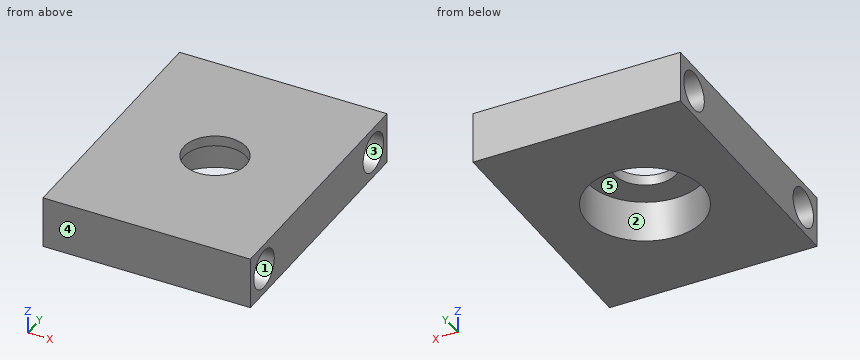
Autodesk Fusion 360 part; units mm, degrees
sketch "Top" plane through (0, 0, 0) normal (0, 0, 1) x (1, 0, 0)
  line L0 (0, 0) -> (40, 0)
  line L1 (40, 0) -> (40, 50)
  line L2 (40, 50) -> (0, 50)
  line L3 (0, 50) -> (0, 0)
  circle A0 centre (20, 25) radius 11.2
  circle A1 centre (20, 25) radius 6
  dimension "d6" = 40
  dimension "d7" = 50
  dimension "d11" = 22.4
  dimension "d12" = 25
  dimension "d13" = 20
  dimension "d27" = 12
extrude "Extrude1" add sketch "Top" along normal blind 10 contours L0 L1 L2 L3 | A0 | A1
extrude "Extrude2" cut sketch "Top" along normal blind 8 contours A0 | A1
sketch "Sketch2" plane through (40, 0, 0) normal (1, 0, 0) x (0, 1, 0)
  line L0 (0, 0) -> (50, 0)
  line L1 (50, 0) -> (50, 10)
  line L2 (50, 10) -> (0, 10)
  line L3 (0, 10) -> (0, 0)
  circle A0 centre (5, 5) radius 3.75
  circle A1 centre (45, 5) radius 3.75
  dimension "d16" = 7.5
  dimension "d17" = 7.5
  dimension "d18" = 5
  dimension "d19" = 5
  dimension "d20" = 5
  dimension "d21" = 5
extrude "Extrude3" cut sketch "Sketch2" against normal blind 50 contours A0
extrude "Extrude4" cut sketch "Sketch2" against normal blind 50 contours A1
extrude "Extrude5" cut sketch "Top" along normal blind 20 contours A1
equation "length = 50 mm"
equation "width = 40 mm"
equation "thickness = 10 mm"
equation "extra = 10 mm"
equation "fit_gap = 0.2 mm"
equation "d6 = width"
equation "d7 = length"
equation "d8 = thickness"
equation "bearing_outer_radius = 11.1 mm"
equation "d11 = ( bearing_outer_radius * 2 ) + fit_gap"
equation "d12 = length / 2"
equation "d13 = width / 2"
equation "d14 = thickness - 2 mm"
equation "d16 = 3 * thickness / 4"
equation "d17 = 3 * thickness / 4"
equation "d18 = thickness / 2"
equation "d19 = thickness / 2"
equation "d20 = thickness / 2"
equation "d21 = thickness / 2"
equation "bearing_inner_radius = ( 8 mm + 4 mm ) / 2"
equation "d27 = bearing_inner_radius * 2"
equation "d28 = thickness + extra"
Check sheet for the modelled part. Datum: model origin and axes. Units: mm. Face numbers are marked on the shaded views. A direction names the side the tool comes from. Round coordinates to 2 decimals unless told otherwise and drop trailing zeros. Order: outer loops, then holes, each group sorted by start corner. A loop starts at its lowest first (then second) coordinate and runs counter-clockwise, first axis right, second up. Notation, with made-up numbers: M -23,16 L 28,16 A20 cw 28,23 Z; hole C -1,24 d7. An arc over 180 degrees is marked long. One line per item, written item: value. Start each with the question number.
1. Section check A-A on x = 20. Enter the section's corners in (y, z), and give its area (3 significant figures).
2. Section check D-D on y = 5. Enter the section's corners in (x, z).
3. Release check for a two-part mould opening along Z. For the marked faces 3, 4 and 5 record: released by +Z, released by -Z, zero draft, split by the parting line, or undercut.
4. Scan lines: line 1 along Y through (x, z) = (8.5, 3.75); line 2 along Z through (x, y) = (13, 5); line 3 along Y through (x, z) = (20, 9.4). Record each from-to range of solid material in increasing order.
5. Section check C-C on z = 5. Enter the section's corners in (x, y), and give its area (3 significant figures).
6. Access from +Z, -Z, +X, -X, +Y, -Y to the whole of each face (thin tool, end or side, straight path). Record for the marked faces 1 and 2.
7. Section check B-B on y = 25. Enter the section's corners in (x, z).
8. Gauge pin test, flat end, axial feed: P1, Ø1, axis at x = 21, y = 33.5, coming from the -Z side. Record the tip position at first contact, or that the pin passes through.
Results found:
1. outline: M 0,0 L 13.8,0 L 13.8,8 L 19,8 L 19,10 L 0,10 Z; M 31,8 L 36.2,8 L 36.2,0 L 50,0 L 50,10 L 31,10 Z; hole C 5,5 d7.5; hole C 45,5 d7.5
1. area: 208 mm^2
2. outline: M 0,0 L 40,0 L 40,1.25 L 0,1.25 Z; M 0,8.75 L 40,8.75 L 40,10 L 0,10 Z
3. face 3: undercut
3. face 4: zero draft
3. face 5: released by -Z
4. line 1: 0 to 1.46, 8.54 to 41.46, 48.54 to 50
4. line 2: 0 to 1.25, 8.75 to 10
4. line 3: 0 to 19, 31 to 50
5. outline: M 0,0 L 40,0 L 40,1.25 L 0,1.25 Z; M 0,8.75 L 40,8.75 L 40,41.25 L 0,41.25 Z; M 0,48.75 L 40,48.75 L 40,50 L 0,50 Z; hole C 20,25 d22.4
5. area: 1,010 mm^2
6. face 1: +X, -X
6. face 2: -Z
7. outline: M 0,0 L 8.8,0 L 8.8,8 L 14,8 L 14,10 L 0,10 Z; M 26,8 L 31.2,8 L 31.2,0 L 40,0 L 40,10 L 26,10 Z
8. P1: z = 8
